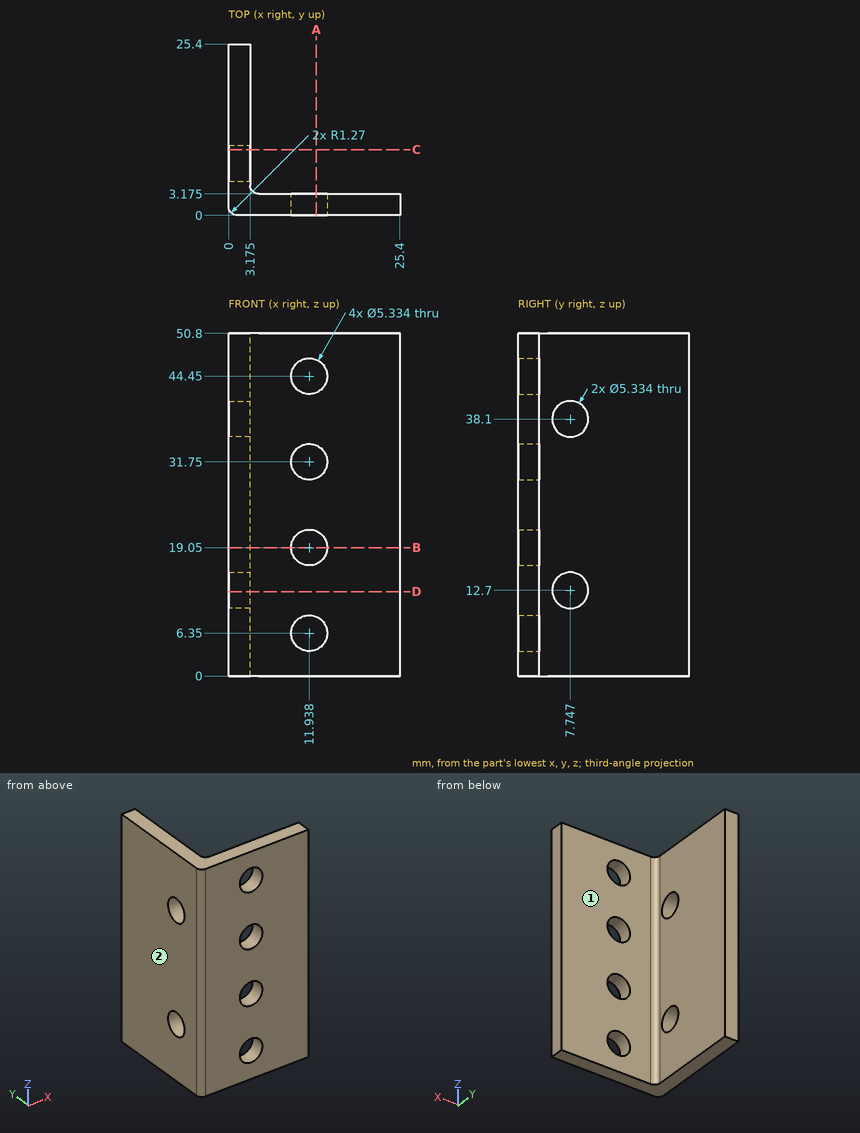
Geometry check sheet. Reference: drawing and pictorial views, mm from the part's lowest x, y, z. A direction names the side the tool comes from. Give positions to 0.01 mm unless a question says otherwise; leave off trailing zeros. Loops run counter-clockwise (first coordinate to the right, second up) from the corner with the lowest first, then second, coordinate; pieces in that order, holes last. Notation, with made-up numbers: (69, -14) - (102, -14) arc R17 cw to (102, -2) - close; hole circle Ø7 at (87, -21.75). An arc over 180 degrees is marked (long way). One line per question, with ' | ' between items. Start each with the question number.
1. Cross-section at A-A, the plane x = 13. Enter the section's corners in (y, z) (3 decimals).
2. Set-up check for the marked faces 1 and 2: record each of +Z, -Z, +X, -X, +Y, -Y from which the full face is reachable in a straight line by a thin tool's end or side.
3. Material ranges on line 1 along X through (y, z) = (2.45, 44.45) (3 decimals); line 2 along Y through (x, z) = (2.5, 12.7); line 3 along Y through (x, z) = (5, 45) (3 decimals), recorded low to high. Write a range as [from, to].
4. Cross-section at C-C, the plane y = 9.75. Enter the section's corners in (x, z) (3 decimals), plus the area to 3 significant figures.
5. Cross-section at B-B, the plane z = 19.05. Enter the section's corners in (x, y) (3 decimals).
6. Cross-section at D-D, the plane z = 12.5. Enter the section's corners in (x, y) (1 decimal).
7. Gauge pin test, flat ends, axial feed: pin 1 Ø1.5 at (x, z) = (17, 27.5) entering from +Y (3 decimals); pin 2 Ø4 at (y, z) = (18, 34) entering from +X (3 decimals). Record the tip position at first contact, or that the pin passes through.
Check result:
1) outline: (0, 0) - (3.175, 0) - (3.175, 3.904) - (0, 3.904) - close; (0, 8.796) - (3.175, 8.796) - (3.175, 16.604) - (0, 16.604) - close; (0, 21.496) - (3.175, 21.496) - (3.175, 29.304) - (0, 29.304) - close; (0, 34.196) - (3.175, 34.196) - (3.175, 42.004) - (0, 42.004) - close; (0, 46.896) - (3.175, 46.896) - (3.175, 50.8) - (0, 50.8) - close
2) face 1: +Z, -Z, +X, +Y | face 2: +Z, -Z, -X, +Y, -Y
3) line 1: x = [0, 9.271], [14.605, 25.4] | line 2: y = [0, 5.08], [10.41, 25.4] | line 3: y = [0, 3.175]
4) outline: (0, 0) - (3.175, 0) - (3.175, 10.939) - (0, 10.939) - close; (0, 14.461) - (3.175, 14.461) - (3.175, 36.339) - (0, 36.339) - close; (0, 39.861) - (3.175, 39.861) - (3.175, 50.8) - (0, 50.8) - close | area: 139 mm2
5) outline: (0, 1.27) arc R1.27 ccw to (1.27, 0) - (9.271, 0) - (9.271, 3.175) - (4.445, 3.175) arc R1.27 cw to (3.175, 4.445) - (3.175, 25.4) - (0, 25.4) - close; (14.605, 0) - (25.4, 0) - (25.4, 3.175) - (14.605, 3.175) - close
6) outline: (0, 1.3) arc R1.3 ccw to (1.3, 0) - (25.4, 0) - (25.4, 3.2) - (4.4, 3.2) arc R1.3 cw to (3.2, 4.4) - (3.2, 5.1) - (0, 5.1) - close; (0, 10.4) - (3.2, 10.4) - (3.2, 25.4) - (0, 25.4) - close
7) pin 1: stops at y = 3.175 | pin 2: stops at x = 3.175
